from build123d import *

# Parameters (mm, degrees)
SKETCH_1_W          = 20
SKETCH_1_H          = 20
EXTRUDE_1_DEPTH     = 245
SKETCH_2_W          = 14
SKETCH_2_H          = 14
CUT_EXTRUDE_1_DEPTH = 246
SKETCH_3_R          = 1.5
SKETCH_3_R_2        = 1.6
CUT_EXTRUDE_2_DEPTH = 80
SKETCH_4_R          = 2.5
CUT_EXTRUDE_3_DEPTH = 93


with BuildPart() as part:
    # 草图1 → 凸台-拉伸1 (new body)
    with BuildSketch(Plane.XY):
        with Locations((0.666666667, 1.006147649)):
            Rectangle(SKETCH_1_W, SKETCH_1_H)
    extrude(amount=EXTRUDE_1_DEPTH)

    # 草图2 → 切除-拉伸1 (cut, through all)
    with BuildSketch(Plane(origin=(0, 0, 0), x_dir=(-1, 0, 0), z_dir=(0, 0, -1))):
        with Locations((-0.666666667, 1.006147649)):
            Rectangle(SKETCH_2_W, SKETCH_2_H)
    extrude(amount=-CUT_EXTRUDE_1_DEPTH, mode=Mode.SUBTRACT)

    # 草图3 → 切除-拉伸2 (cut)
    with BuildSketch(Plane.ZY.offset(9.333333333)):
        with Locations((225, 1.006147649)):
            Circle(SKETCH_3_R)
        with Locations((195, 1.006147649)):
            Circle(SKETCH_3_R)
        with Locations((165, 1.006147649)):
            Circle(SKETCH_3_R)
        with Locations((20, 1.006147649)):
            Circle(SKETCH_3_R_2)
    extrude(amount=-CUT_EXTRUDE_2_DEPTH, mode=Mode.SUBTRACT)

    # 草图4 → 切除-拉伸3 (cut)
    with BuildSketch(Plane(origin=(0, 11.006147649, 0), x_dir=(1, 0, 0), z_dir=(0, 1, 0))):
        with Locations((0.666666667, -17.788232679)):
            Circle(SKETCH_4_R)
        with Locations((0.666666667, -81.833059371)):
            Circle(SKETCH_4_R)
        with Locations((0.666666667, -163.166940629)):
            Circle(SKETCH_4_R)
        with Locations((0.666666667, -227.211767321)):
            Circle(SKETCH_4_R)
    extrude(amount=-CUT_EXTRUDE_3_DEPTH, mode=Mode.SUBTRACT)


solid = part.part
Geometry: final body of the model. Coordinates: model frame, mm. A direction names the side the tool comes from. Give positions to 0.01 mm unless a question says otherwise; leave off trailing zeros. Loops run counter-clockwise (first coordinate to the right, second up) from the corner with the lowest first, then second, coordinate; pieces in that order, holes last. Notation, with made-up numbers: M -3.75,-23.5 L 49.25,-23.5 A29 cw 49.25,0.5 Z; hole C 47.5,82 d6. An arc over 180 degrees is marked long. Put each result on its own line as item: value. Start each with the question number.
1) Contact query for a flat-ended pin moving along its axis: pin 1 (3.5 mm diameter, centred on y = 1.01, z = 195, fed in from +X). Output: stop coordinate, or through.
2) Ray query, line 1 along Y through (x, z) = (-1, 69); line 2 along Y through (x, z) = (-8.15, 195); line 3 along X through (y, z) = (4, 93). Return the intervals inside material, ascending.
3) Cut plane B-B (z = 68.5). Output: boundary loops of the cut face in (x, y).
4) Access query for faces 4 (the cylindrical face through (0.12, -7.47, 229.65)), 5 (the flat face through (1, -5.994, 121)). Directions: +Z, -Z, +X, -X, +Y, -Y. A direction counts if a zero-diameter tool reaches every point of the face in a straight line with its end or side. Return the directions, or none.
5) Pull-direction query (X, two-part tool) for faces 1 (the flat face through (-8, 1, 0)), 2 (the cylindrical face through (2.01, 9.53, 161.06)), 3 (the flat face through (-9.333, 1, 121)); classes: pulls with the +X half, pulls with the -X half, needs draft (parallel to the pull), parting line crosses it, or undercut.
6) Cut plane A-A (y = -3). Output: boundary loops of the cut face in (x, z).
Verdict:
1. pin 1: x = 10.67
2. line 1: -8.99 to -5.99, 8.01 to 11.01
2. line 2: -8.99 to -0.49, 2.51 to 11.01
2. line 3: -9.33 to -6.33, 7.67 to 10.67
3. outline: M -9.33,-8.99 L 10.67,-8.99 L 10.67,11.01 L -9.33,11.01 Z; hole M -6.33,-5.99 L 7.67,-5.99 L 7.67,8.01 L -6.33,8.01 Z
4. face 4: +Y, -Y
4. face 5: +Z, -Z
5. face 1: needs draft
5. face 2: undercut
5. face 3: pulls with the -X half
6. outline: M -9.33,0 L -6.33,0 L -6.33,245 L -9.33,245 Z; M 7.67,0 L 10.67,0 L 10.67,245 L 7.67,245 Z
